```python
from build123d import *

# Parameters (mm, degrees)
SKETCH2_R                           = 1.725862242
BOSS_EXTRUDE1_DEPTH                 = 5.08
CIRPATTERN1_COUNT                   = 4
TAP_DRILL_FOR_1_12_TAP1_D           = 23.41626
TAP_DRILL_FOR_1_12_TAP1_CSINK_D     = 24.68626
TAP_DRILL_FOR_1_12_TAP1_CSINK_ANGLE = 100
CIRPATTERN2_COUNT                   = 4
SKETCH4_R                           = 3.927379396
CUT_EXTRUDE1_DEPTH                  = 205.678906094
CIRPATTERN3_COUNT                   = 2


with BuildPart() as part:
    # Sketch1 → Revolve1 (revolve)
    with BuildSketch(Plane.XY, mode=Mode.PRIVATE) as revolve1_sk:
        Polygon((-75.276594545, 31.75), (-75.276594545, 67.5005), (-26.279994545, 67.5005), (-26.279994545, 113.4999), (51.723405455, 113.4999), (51.723405455, 53.34), (51.723405455, 36.268932417), (59.730205455, 36.268932417), (59.730205455, 57.15), (80.730205455, 57.15), (80.730205455, 31.75), align=None)
    revolve(revolve1_sk.sketch.rotate(Axis((-77.058289091, 0, 0), (1, 0, 0)), 90), axis=Axis((-77.058289091, 0, 0), (1, 0, 0)))

    # Sketch2 → Boss-Extrude1 (add)
    with BuildSketch(Plane(origin=(51.723405455, 0, 0), x_dir=(0, 0, -1), z_dir=(1, 0, 0))):
        with BuildLine():
            Line((9.502237171, 69.200650205), (9.502237171, 77.59727245))
            ThreePointArc((9.502237171, 77.59727245), (-0.022762829, 81.693250486), (-9.547762829, 77.59727245))
            Line((-9.547762829, 77.59727245), (-9.547762829, 69.194383623))
            Line((-9.547762829, 69.194383623), (-9.547762829, 40.334566498))
            Line((-9.547762829, 40.334566498), (9.502237171, 40.334566498))
            Line((9.502237171, 40.334566498), (9.502237171, 69.200650205))
        make_face()
        with Locations((0, 74.333669045)):
            Circle(SKETCH2_R, mode=Mode.SUBTRACT)
    boss_extrude1 = extrude(amount=BOSS_EXTRUDE1_DEPTH)

    # CirPattern1: Boss-Extrude1 ×4 about axis
    cirpattern1_axis = Axis((0, 0, 0), (1, 0, 0))
    for i in range(1, CIRPATTERN1_COUNT):
        add(boss_extrude1.rotate(cirpattern1_axis, i * 360 / CIRPATTERN1_COUNT))

    # Tap Drill for 1-12 Tap1 (through all)
    with Locations(Plane(origin=(51.723405455, 67.172315786, 67.172315786), x_dir=(0, 0, 1), z_dir=(1, 0, 0))):
        with Locations((0, 0)):
            tap_drill_for_1_12_tap1 = CounterSinkHole(TAP_DRILL_FOR_1_12_TAP1_D / 2, TAP_DRILL_FOR_1_12_TAP1_CSINK_D / 2, counter_sink_angle=TAP_DRILL_FOR_1_12_TAP1_CSINK_ANGLE)

    # CirPattern2: Tap Drill for 1-12 Tap1 ×4 about axis
    cirpattern2_axis = Axis((0, 0, 0), (1, 0, 0))
    for i in range(1, CIRPATTERN2_COUNT):
        add(tap_drill_for_1_12_tap1.rotate(cirpattern2_axis, i * 360 / CIRPATTERN2_COUNT), mode=Mode.SUBTRACT)

    # Sketch4 → Cut-Extrude1 (cut, through all)
    with BuildSketch(Plane(origin=(51.723405455, 0, 0), x_dir=(0, 0, -1), z_dir=(1, 0, 0))):
        with Locations((-89.48120145, -31.895996663)):
            Circle(SKETCH4_R)
    cut_extrude1 = extrude(amount=-CUT_EXTRUDE1_DEPTH, mode=Mode.SUBTRACT)

    # CirPattern3: Cut-Extrude1 ×2 about axis
    cirpattern3_axis = Axis((0, 0, 0), (1, 0, 0))
    for i in range(1, CIRPATTERN3_COUNT):
        add(cut_extrude1.rotate(cirpattern3_axis, i * 360 / CIRPATTERN3_COUNT), mode=Mode.SUBTRACT)


solid = part.part
```
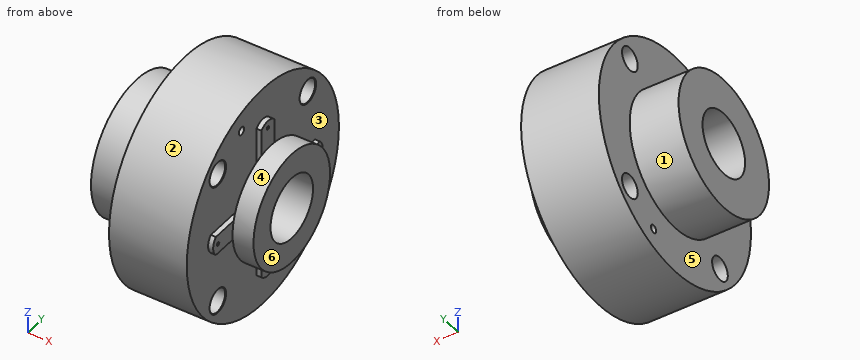
Check sheet for the modelled part. Datum: model origin and axes. Units: mm. Face numbers are marked on the shaded views. A direction names the side the tool comes from. Give positions to 0.01 mm unless a question says otherwise; leave off trailing zeros. Order: outer loops, then holes, each group sorted by start corner. A loop starts at its lowest first (then second) coordinate and runs counter-clockwise, first axis right, second up. Notation, with made-up numbers: M 78.25,19.25 L 100.25,19.25 A14 ccw 100.25,37.25 Z; hole C 13.25,-30 d1. An arc over 180 degrees is marked long. Answer in a Markdown table with one row per item.
1) Access from +Z, -Z, +X, -X, +Y, -Y to the whole of each face (thin tool, end or side, straight path). Record for the marked faces 1 and 2.
Filled sheet:
| item | result |
|---|---|
| face 1 | -X |
| face 2 | +X, -X |
2) Cross-section at D-D, the plane x = -40.5. Enter the section's corners in (y, z), plus the area to 3 significant figures.
Filled sheet:
| item | result |
|---|---|
| outline | C 0,0 d135; hole C 0,0 d63.5 |
| area | 11,100 mm2 |
3) Cross-section at A-A, the plane y = 21.5. Enter the section's corners in (x, z).
Filled sheet:
| item | result |
|---|---|
| outline | M -75.28,-63.98 L -26.28,-63.98 L -26.28,-111.44 L 51.72,-111.44 L 51.72,-29.21 L 59.73,-29.21 L 59.73,-52.95 L 80.73,-52.95 L 80.73,-23.36 L -75.28,-23.36 Z; M -75.28,23.36 L 80.73,23.36 L 80.73,52.95 L 59.73,52.95 L 59.73,29.21 L 51.72,29.21 L 51.72,111.44 L -26.28,111.44 L -26.28,63.98 L -75.28,63.98 Z |
4) Release check for a two-part mould opening along X. For the marked faces 3, 4, 5 and 6 record: +X half, -X half, draft (parallel to the pull), parting line (faces both ways), or undercut.
Filled sheet:
| item | result |
|---|---|
| face 3 | undercut |
| face 4 | draft |
| face 5 | -X half |
| face 6 | +X half |
5) Cross-section at C-C, the plane x = 45. Enter the section's corners in (y, z).
Filled sheet:
| item | result |
|---|---|
| outline | C 0,0 d227; hole C -67.17,-67.17 d23.42; hole C -67.17,67.17 d23.42; hole C -31.9,89.48 d7.85; hole C 0,0 d63.5; hole C 31.9,-89.48 d7.85; hole C 67.17,-67.17 d23.42; hole C 67.17,67.17 d23.42 |
6) Gauge pin test, flat ends, axial feed: P1, Ø4, axis at y = -74.5, z = -0.5, coming from the +X side; P2, Ø8, axis at y = -74, z = 32, coming from the -X side; P3, Ø3, axis at x = -50.5, z = -48, coming from the +Y side; P4, Ø14, axis at y = 67.17, z = 67.17, coming from the -X side. Record the tip position at first contact, or that the pin passes through.
Filled sheet:
| item | result |
|---|---|
| P1 | stops at x = 56.8 |
| P2 | stops at x = -26.28 |
| P3 | stops at y = 48.93 |
| P4 | passes through |
7) Thickness scan on L1, parallel to Y at x = -13, z = 76.5; L2, parallel to X at y = 27, z = -24.5; L3, parallel to Y at x = 32, z = 72. Record the ranges inside material, lowest first. Write a range as [from, to].
Filled sheet:
| item | result |
|---|---|
| L1 | y = [-83.84, -74.25], [-60.1, 60.1], [74.25, 83.84] |
| L2 | x = [-75.28, 51.72], [59.73, 80.73] |
| L3 | y = [-87.74, -77.84], [-56.51, 56.51], [77.84, 87.74] |
8) Cross-section at B-B, the plane z = -24.5. Enter the section's corners in (x, y), plus the area to 3 significant figures.
Filled sheet:
| item | result |
|---|---|
| outline | M -75.28,-62.9 L -26.28,-62.9 L -26.28,-110.82 L 51.72,-110.82 L 51.72,-26.74 L 59.73,-26.74 L 59.73,-51.63 L 80.73,-51.63 L 80.73,-20.19 L -75.28,-20.19 Z; M -75.28,20.19 L 80.73,20.19 L 80.73,51.63 L 59.73,51.63 L 59.73,26.74 L 51.72,26.74 L 51.72,110.82 L -26.28,110.82 L -26.28,62.9 L -75.28,62.9 Z |
| area | 19,700 mm2 |
